Autodesk Inventor part; units mm, degrees
ref_plane "Work Plane9" through (82.5476, 165.0953, 0) normal (0.5773503, 0.5773503, 0.5773503) x (0.7071068, 0, -0.7071068)
ref_plane "YZ Plane" through (0, 0, 0) normal (1, 0, 0) x (0, 1, 0)
ref_plane "XZ Plane" through (0, 0, 0) normal (0, 1, 0) x (-1, 0, 0)
sketch "Sketch26" plane through (0, 0, 0) normal (0, 0, 1) x (1, 0, 0)
  line L0 (82.5476, 0) -> (0, 82.5476)
  line L1 (0, 82.5476) -> (-82.5476, 0)
  line L2 (-82.5476, 0) -> (0, -82.5476)
  line L3 (0, -82.5476) -> (82.5476, 0)
  line L4 (-58.37, -58.37) -> (58.37, 58.37) construction
  line L5 (58.37, -58.37) -> (-58.37, 58.37) construction
  point P0 (0, 0)
  dimension "d97" = 116.74
  dimension "d98" = 165.0953
extrude "Extrusion9" add sketch "Sketch26" along normal mid plane 330.1906
pattern_circular "Circular Pattern14" count 4 over 360 about axis through (-10, 0, 0) along (1, 0, 0) of "Extrusion9"
pattern_circular "Circular Pattern15" count 4 over 360 about axis through (0, -10, 0) along (0, 1, 0) of "Extrusion9"
ref_plane "Work Plane9" through (82.5476, 165.0953, 0) normal (0.5773503, 0.5773503, 0.5773503) x (0.7071068, 0, -0.7071068)
sketch "Sketch27" plane through (82.5476, 165.0953, 0) normal (0.5773503, 0.5773503, 0.5773503) x (0.7071068, 0, -0.7071068)
  line L0 (-116.74, -67.3999) -> (-116.74, 0)
  line L1 (-116.74, 0) -> (0, 0)
  line L2 (0, 0) -> (58.37, -101.0998)
  line L3 (58.37, -101.0998) -> (0, -202.1996)
  line L4 (0, -202.1996) -> (-116.74, -202.1996)
  line L5 (-116.74, -202.1996) -> (-175.11, -101.0998)
  line L6 (-175.11, -101.0998) -> (-116.74, 0)
  point P0 (-58.37, -101.0998)
  point P1 (-58.37, -101.0998)
extrude "Extrusion10" add sketch "Sketch27" against normal up to surface (285.9534 mm away)
pattern_circular "Circular Pattern16" count 4 over 360 about axis through (-10, 0, 0) along (1, 0, 0) of "Extrusion10"
shell "Shell2" thickness 5 removed faces 1 at (0, -165.0953, -27.5159)
equation "\"d99\" = 2 * d98"
equation "\"d107\" = 2 * d98"
properties part number "Dome" material "Glass"
CAD build for the part. Positions are in the model's coordinates, mm. A direction names the side the tool comes from. Round coordinates to 2 decimals unless told otherwise and drop trailing zeros. Loops run counter-clockwise (first coordinate to the right, second up) from the corner with the lowest first, then second, coordinate; pieces in that order, holes last. Notation, with made-up numbers: M 1.5,-14 L 43.5,-14 A14 ccw 43.5,5 Z; hole C -4.75,-10 d5. An arc over 180 degrees is marked long. Return JSON: item names as keys, results as strings. Group by question number.
(1) Saw through at D-D, the plane x = 17. List the corners of the cut face in (y, z).
(2) Saw through at A-A, the plane x = -90. List the corners of the cut face in (y, z).
(3) Mould opens along Y. For faces 3 (the flat face through (-84.28, -81.39, -81.97)), 4 (the flat face through (80.81, 83.7, 83.13)), 5 (the flat face through (77.786, 80.028, -81.168)) say: +Y half, -Y half, draft (parallel to the pull), parting line (faces both ways), or undercut.
(4) Drop flat-ended pins along their axis: P1, Ø12, axis at x = -42.5, y = -100.5, coming from the +Z side; P2, Ø2, axis at y = 109.5, z = 128.5, coming from the -X side; P3, Ø8, axis at x = -16.5, z = -116, coming from the +Y side. Give the stop position or say it passes through.
(5) Saw through at B-B, the plane y = 68.5. List the corners of the cut face in (x, z).
(6) Saw through at C-C, the plane z = 143.5. List the corners of the cut face in (x, y), and give its area (3 significant figures).
(7) Wall check: probe 1 along X at (y, z) = (41.5, -10); probe 2 along Z at (x, y) = (-63, 93). Give the ranges that are in metal, low to high. Write a range as [from, to].
(8) Tool access for faces 1 (the flat face through (-165.095, 1, 1)), 2 (the flat face through (-81.149, 78.927, 78.907)): list every direction of +Z, -Z, +X, -X, +Y, -Y with a clear straight run to the whole face (end or side of a thin tool).
Answer list:
{
 "1": {"outline": "M -165.1,-65.55 L -65.55,-165.1 L 65.55,-165.1 L 165.1,-65.55 L 165.1,65.55 L 65.55,165.1 L -65.55,165.1 L -165.1,65.55 L -165.1,56.89 L -61.89,160.1 L 61.89,160.1 L 160.1,61.89 L 160.1,-61.89 L 61.89,-160.1 L -61.89,-160.1 L -165.1,-56.89 Z"},
 "2": {"outline": "M -157.64,0 L 0,-157.64 L 157.64,0 L 0,157.64 Z; hole M -148.98,0 L 0,-148.98 L 148.98,0 L 0,148.98 Z"},
 "3": {"face 3": "-Y half", "face 4": "+Y half", "face 5": "undercut"},
 "4": {"P1": "z = 113.13", "P2": "x = -11.06", "P3": "y = 120.8"},
 "5": {"outline": "M -165.1,-14.05 L -14.05,-165.1 L 14.05,-165.1 L 165.1,-14.05 L 165.1,14.05 L 14.05,165.1 L -14.05,165.1 L -165.1,14.05 Z; hole M -160.1,-10.39 L -10.39,-160.1 L 10.39,-160.1 L 160.1,-10.39 L 160.1,10.39 L 10.39,160.1 L -10.39,160.1 L -160.1,10.39 Z"},
 "6": {"outline": "M -104.14,0 L 0,-104.14 L 104.14,0 L 0,104.14 Z; hole M -95.48,0 L 0,-95.48 L 95.48,0 L 0,95.48 Z", "area": "3,460 mm2"},
 "7": {"probe 1": "[-165.1, -160.1], [160.1, 165.1]", "probe 2": "[-91.64, -82.98], [82.98, 91.64]"},
 "8": {"face 1": "+Z, -Z, -X, +Y, -Y", "face 2": "none"}
}
